Part model, mm, in its own coordinate system. A direction names the side the tool comes from. Coordinates: 2 decimals unless noted, no trailing zeros. Use a Markdown table: item, result.
```python
from build123d import *

# Parameters (mm, degrees)
BOSS_EXTRUDE1_DEPTH = 12
SKETCH2_W           = 2.8
SKETCH2_H           = 7.3
CUT_EXTRUDE1_DEPTH  = 10


with BuildPart() as part:
    # Sketch1 → Boss-Extrude1 (new body)
    with BuildSketch(Plane.XY):
        with BuildLine():
            Line((5, 0), (59, 0))
            ThreePointArc((59, 0), (62.535533906, 1.464466094), (64, 5))
            Line((64, 5), (64, 113))
            ThreePointArc((64, 113), (62.535533906, 116.535533906), (59, 118))
            Line((59, 118), (5, 118))
            ThreePointArc((5, 118), (1.464466094, 116.535533906), (0, 113))
            Line((0, 113), (0, 5))
            ThreePointArc((0, 5), (1.464466094, 1.464466094), (5, 0))
        make_face()
    extrude(amount=-BOSS_EXTRUDE1_DEPTH)

    # Sketch2 → Cut-Extrude1 (cut)
    with BuildSketch(Plane(origin=(0, 0, 0), x_dir=(0, 0, -1), z_dir=(1, 0, 0))):
        with Locations((6, 32.5)):
            Rectangle(SKETCH2_W, SKETCH2_H)
    extrude(amount=CUT_EXTRUDE1_DEPTH, mode=Mode.SUBTRACT)


solid = part.part
```
Item 1: Drill centre lines: probe 1 along Z at (x, y) = (7.5, 32.5); probe 2 along X at (y, z) = (31, -6.25); probe 3 along Y at (x, z) = (61, -9.5). Where is each one in solid material? Low to high.
From the geometry:
| item | result |
|---|---|
| probe 1 | -12 to -7.4, -4.6 to 0 |
| probe 2 | 10 to 64 |
| probe 3 | 0.42 to 117.58 |
Item 2: Which spindle directions (+Z, -Z, +X, -X, +Y, -Y) get a long thin tool onto all of the face, cutting with end or side? Do faces 1 (the face through (5, 32, -7.4)), 2 (the face through (62, 1, -6)). Say none if no direction does.
From the geometry:
| item | result |
|---|---|
| face 1 | -X |
| face 2 | +Z, -Z, +X, -Y |
Item 3: Drop a flat-ended pin along its axis: P1, Ø0.8, axis at x = 3.5, z = -5.5, coming from the -Y side. Give the stop position or say it passes through.
From the geometry:
| item | result |
|---|---|
| P1 | y = 0.12 |
Item 4: Two-plate mould, pull along Y, no slides. Class faces 3 (the face through (64, 58, -6)), 4 (the face through (63, 116, -6)), 5 (the face through (10, 33, -6)): pulls with the +Y half, pulls with the -Y half, needs draft (parallel to the pull), parting line crosses it, or undercut.
From the geometry:
| item | result |
|---|---|
| face 3 | needs draft |
| face 4 | pulls with the +Y half |
| face 5 | undercut |
